The listing builds one solid part. Answer for the finished solid, in the listing's coordinates (mm). A direction names the side the tool comes from. Round coordinates to 2 decimals unless told otherwise and drop trailing zeros. Write each loop counter-clockwise with the first axis right and the second up, starting at its lowest first coordinate (ties: lowest second). Pieces come first, ordered by that corner, then holes.
(1) A cutting plane is placed at D-D, the plane y = -1.5. Give the vertices of the cut face in (x, z), and give its area (3 significant figures).
(2) Each of these flat-tipped pins is pushed along its axis until it touches: pin 1 Ø3 at (x, y) = (12, -5.5) entering from +Z; pin 2 Ø3 at (x, z) = (8, 4.5) entering from -Y; pin 3 Ø1.5 at (x, z) = (11, 1) entering from -Y. Where does it stop, or does it pass through?
(3) A cutting plane is placed at B-B, the plane y = -5. Give the vertices of the cut face in (x, z), and give its area (3 significant figures).
(4) Find the intervals of material crossed by probe 1 along Z at (x, y) = (9.5, -5.25); probe 2 along Y at (x, z) = (13, -0.45), in increasing order.
(5) For faces 4 (the face through (0, -5, -1)), 5 (the face through (9, -2, 2)), determine the directions among +Z, -Z, +X, -X, +Y, -Y from which every point of the face is accessible in a straight line to the end or side of a thin tool.
(6) The mould has two halves that part along Z. Classify faces 1 (the face through (9.126, -0.823, -1.22)), 2 (the face through (11.5, -4.93, -0.99)), 3 (the face through (7.67, -1.01, 3.31)): +Z half, -Z half, draft (parallel to the pull), parting line (faces both ways), or undercut.
(7) A cutting plane is placed at C-C, the plane z = 4.25. Give the vertices of the cut face in (x, y).
(8) A cutting plane is placed at A-A, the plane x = 9. Give the vertices of the cut face in (y, z), and give its area (3 significant figures).
from build123d import *

# Parameters (mm, degrees)
SKETCH_1_W                       = 18
SKETCH_1_H                       = 9
SKETCH_1_R                       = 1.5
SM_BASE_FLANGE_1_DEPTH           = 2
SM_EDGE_FLANGE_1_STRIP_W         = 9.4732
SM_EDGE_FLANGE_1_STRIP_H         = 2
SM_EDGE_FLANGE_1_STRIP_CUT_DEPTH = 18
SM_EDGE_FLANGE_1_DEPTH           = 18
SKETCH_9_R                       = 1.5
CUT_EXTRUDE_1_DEPTH              = 10


# Sheet-metal steps are written as plain solids
with BuildPart() as part:
    # Sketch 1 → 基体-法兰1 (new body)
    with BuildSketch(Plane.XY):
        with Locations((9, -4.5)):
            Rectangle(SKETCH_1_W, SKETCH_1_H)
        with Locations((5, -5)):
            Circle(SKETCH_1_R, mode=Mode.SUBTRACT)
        with Locations((13, -5)):
            Circle(SKETCH_1_R, mode=Mode.SUBTRACT)
    extrude(amount=-SM_BASE_FLANGE_1_DEPTH)

    # 边线-法兰1 strip (across the edge) → 边线-法兰1 strip cut (cut)
    with BuildSketch(Plane(origin=(18, 0, 0), x_dir=(0, -1, 0), z_dir=(-1, 0, 0))):
        with Locations((-2, -1)):
            Rectangle(SM_EDGE_FLANGE_1_STRIP_W, SM_EDGE_FLANGE_1_STRIP_H)
    extrude(amount=SM_EDGE_FLANGE_1_STRIP_CUT_DEPTH, mode=Mode.SUBTRACT)

    # 边线-法兰1 section (across the edge) → 边线-法兰1 (add)
    with BuildSketch(Plane(origin=(18, 0, 0), x_dir=(0, -1, 0), z_dir=(-1, 0, 0))):
        with BuildLine():
            Line((0, 0.7366), (0, 18))
            Line((0, 18), (2, 18))
            Line((2, 18), (2, 0.7366))
            ThreePointArc((2, 0.7366), (2.215745145, 0.215745145), (2.7366, 0))
            Line((2.7366, 0), (2.7366, -2))
            ThreePointArc((2.7366, -2), (0.801531583, -1.198468417), (0, 0.7366))
        make_face()
    extrude(amount=SM_EDGE_FLANGE_1_DEPTH)

    # 草图9 → 切除-拉伸1 (cut)
    with BuildSketch(Plane.XZ.offset(2)):
        with Locations(Location((9, 4, 0), (0, 0, 270))):
            Circle(SKETCH_9_R)
        with BuildLine():
            Line((18, 0.7366), (18, 18))
            Line((18, 18), (0, 18))
            Line((0, 18), (0, 0.7366))
            ThreePointArc((0, 0.7366), (9, 7.5), (18, 0.7366))
        make_face()
    extrude(amount=-CUT_EXTRUDE_1_DEPTH, mode=Mode.SUBTRACT)


solid = part.part
Solutions:
1. outline: (0, -1.7) - (18, -1.7) - (18, 0.74) arc R9.37 ccw to (0, 0.74) - close; hole circle Ø3 at (9, 4)
1. area: 127 mm2
2. pin 1: stops at z = 0
2. pin 2: stops at y = -2
2. pin 3: stops at y = -2.18
3. outline: (0, -2) - (3.5, -2) - (3.5, 0) - (0, 0) - close; (6.5, -2) - (11.5, -2) - (11.5, 0) - (6.5, 0) - close; (14.5, -2) - (18, -2) - (18, 0) - (14.5, 0) - close
3. area: 24.0 mm2
4. probe 1: z = -2 to 0
4. probe 2: y = -9 to -6.5, -3.5 to -0.27
5. face 4: +Z, -Z, -X, +Y, -Y
5. face 5: +Z, +X, -X, -Y
6. face 1: -Z half
6. face 2: draft
6. face 3: undercut
7. outline: (1.9, -2) - (7.52, -2) - (7.52, 0) - (1.9, 0) - close; (10.48, -2) - (16.1, -2) - (16.1, 0) - (10.48, 0) - close
8. outline: (-9, -2) - (-2.74, -2) arc R2.74 ccw to (0, 0.74) - (0, 2.5) - (-2, 2.5) - (-2, 0.74) arc R0.74 cw to (-2.74, 0) - (-9, 0) - close; (-2, 5.5) - (0, 5.5) - (0, 7.5) - (-2, 7.5) - close
8. area: 25.5 mm2
